Geometry check sheet. Reference: the model listing, model coordinates, mm. A direction names the side the tool comes from. Round coordinates to 2 decimals unless told otherwise and drop trailing zeros. Order: outer loops, then holes, each group sorted by start corner. A loop starts at its lowest first (then second) coordinate and runs counter-clockwise, first axis right, second up. Notation, with made-up numbers: (-26, -6.75) -> (-9, -6.75) arc R38 cw to (-9, 32.25) -> close; hole circle Ø4 at (51, 46.25). An arc over 180 degrees is marked (long way). Use a Markdown table: item, result. Add a question column.
Item 1: Sectioned sample at B-B, the plane x = 0.25. Record the cut outline in (y, z).
Item 2: Mould release check, pull along X, two halves, no side actions. Record for faces 1 (the flat face through (-7, 0, 0)), 2 (the flat face through (6.5, 0, 177)), 3 (the flat face through (-7.5, 0, 177)): pulls with the +X half, pulls with the -X half, needs draft (parallel to the pull), parting line crosses it, or undercut.
Item 3: Material ranges on probe 1 along X at (y, z) = (4.75, 281); probe 2 along Z at (x, y) = (7.05, 0), recorded low to high. Write a range as [from, to].
Item 4: Sectioned sample at A-A, the plane z = 73.5. Record the cut outline in (x, y).
Item 5: Set-up check for faces 4 (the flat face through (0, 6.5, 177)), 5 (the flat face through (7.5, 0, 177)): record each of +Z, -Z, +X, -X, +Y, -Y from which the full face is reachable in a straight line by a thin tool's end or side.
Item 6: Gauge pin test, flat end, axial feed: pin 1 Ø1.5 at (x, y) = (5.5, 0) entering from -Z. Record the tip position at first contact, or that the pin passes through.
from build123d import *

# Parameters (mm, degrees)
SKETCH_1_W          = 15
SKETCH_1_H          = 15
SKETCH_1_W_2        = 13
SKETCH_1_H_2        = 13
EXTRUDE_1_DEPTH     = 360
SKETCH_2_R          = 1.5
CUT_EXTRUDE_1_DEPTH = 25


with BuildPart() as part:
    # 草图1 → 凸台-拉伸1 (new body)
    with BuildSketch(Plane.XY):
        Rectangle(SKETCH_1_W, SKETCH_1_H)
        Rectangle(SKETCH_1_W_2, SKETCH_1_H_2, mode=Mode.SUBTRACT)
    extrude(amount=EXTRUDE_1_DEPTH)

    # 草图2 → 切除-拉伸1 (cut)
    with BuildSketch(Plane.ZY.offset(7.5)):
        with Locations(Location((10, 0, 0), (0, 0, 270))):
            Circle(SKETCH_2_R)
    extrude(amount=-CUT_EXTRUDE_1_DEPTH, mode=Mode.SUBTRACT)


solid = part.part
Found:
| question | item | result |
|---|---|---|
| 1 | outline | (-7.5, 0) -> (-6.5, 0) -> (-6.5, 360) -> (-7.5, 360) -> close; (6.5, 0) -> (7.5, 0) -> (7.5, 360) -> (6.5, 360) -> close |
| 2 | face 1 | needs draft |
| 2 | face 2 | undercut |
| 2 | face 3 | pulls with the -X half |
| 3 | probe 1 | x = [-7.5, -6.5], [6.5, 7.5] |
| 3 | probe 2 | z = [0, 8.5], [11.5, 360] |
| 4 | outline | (-7.5, -7.5) -> (7.5, -7.5) -> (7.5, 7.5) -> (-7.5, 7.5) -> close; hole (-6.5, -6.5) -> (6.5, -6.5) -> (6.5, 6.5) -> (-6.5, 6.5) -> close |
| 5 | face 4 | +Z, -Z |
| 5 | face 5 | +Z, -Z, +X, +Y, -Y |
| 6 | pin 1 | passes through |
